Here's how the part is built. I have some questions about the finished solid (model axes, mm). A direction names the side the tool comes from. Round coordinates to 2 decimals unless told otherwise and drop trailing zeros. Order: outer loops, then holes, each group sorted by start corner. A loop starts at its lowest first (then second) coordinate and runs counter-clockwise, first axis right, second up.
```python
from build123d import *

# Parameters (mm, degrees)
F1_DEPTH  = 40
F2_R      = 5
F3_R      = 2.15
F4_DEPTH  = 25
F5_W      = 4.5
F5_H      = 10
F6_DEPTH  = 58.601
F7_R      = 2.24999
F8_W      = 40
F8_H      = 21.2
F9_DEPTH  = 2.4
F10_W     = 40
F10_H     = 21.2
F11_DEPTH = 2.4
F12_W     = 4.3
F12_H     = 9.6518629789
F13_DEPTH = 10


# Not quite as in the source:
# - a fillet or chamfer is up to 0.001 mm smaller than in the source, because OpenCascade refuses the exact size


with BuildPart() as f1:
    # F0 (on Front) → F1 (new body)
    with BuildSketch(Plane.XZ):
        Polygon((25.3, -18.75), (29.3, -18.75), (29.3, 18.75), (-29.3, 18.75), (-29.3, -18.75), (-25.3, -18.75), (-25.3, 14.75), (25.3, 14.75), align=None)
    extrude(amount=F1_DEPTH)

    # F2
    f2_edges = [f1.edges().sort_by_distance(p)[0] for p in [
        (-29.3, -20, 18.75),
        (29.3, -20, 18.75),
    ]]
    fillet(f2_edges, radius=F2_R)

    # F3 (on face) → F4 (cut)
    with BuildSketch(Plane.XY.offset(18.75)):
        with Locations((0, -20)):
            Circle(F3_R)
    extrude(amount=-F4_DEPTH, mode=Mode.SUBTRACT)

    # F5 (on face) → F6 (cut, through all)
    with BuildSketch(Plane.YZ.offset(29.3)):
        with Locations((-20, -9.25)):
            Rectangle(F5_W, F5_H)
    extrude(amount=-F6_DEPTH, mode=Mode.SUBTRACT)

    # F7 (radius 2.25 in the source; OpenCascade refuses exactly that, so slightly less here)
    f7_edges = [f1.edges().sort_by_distance(p)[0] for p in [
        (27.3, -17.75, -4.25),
        (27.3, -22.25, -4.25),
        (27.3, -17.75, -14.25),
        (27.3, -22.25, -14.25),
        (-27.3, -17.75, -4.25),
        (-27.3, -17.75, -14.25),
        (-27.3, -22.25, -4.25),
        (-27.3, -22.25, -14.25),
    ]]
    fillet(f7_edges, radius=F7_R)

    # F8 (on face) → F9 (join)
    with BuildSketch(Plane(origin=(25.3, 0, 0), x_dir=(0, -1, 0), z_dir=(-1, 0, 0))):
        with Locations((20, -8.15)):
            Rectangle(F8_W, F8_H)
        with BuildLine():
            ThreePointArc((17.75, -6.5), (20, -4.25), (22.25, -6.5))
            Line((22.25, -6.5), (22.25, -12))
            ThreePointArc((22.25, -12), (20, -14.25), (17.75, -12))
            Line((17.75, -12), (17.75, -6.5))
        make_face(mode=Mode.SUBTRACT)
    extrude(amount=F9_DEPTH)

    # F10 (on face) → F11 (join)
    with BuildSketch(Plane.YZ.offset(-25.3)):
        with Locations((-20, -8.15)):
            Rectangle(F10_W, F10_H)
        with BuildLine():
            ThreePointArc((-22.25, -6.5), (-20, -4.25), (-17.75, -6.5))
            Line((-17.75, -6.5), (-17.75, -12))
            ThreePointArc((-17.75, -12), (-20, -14.25), (-22.25, -12))
            Line((-22.25, -12), (-22.25, -6.5))
        make_face(mode=Mode.SUBTRACT)
    extrude(amount=F11_DEPTH)

    # F12 (on face) → F13 (join)
    with BuildSketch(Plane(origin=(0, 0, 14.75), x_dir=(1, 0, 0), z_dir=(0, 0, -1))):
        with Locations((0, 35.1740685105)):
            Rectangle(F12_W, F12_H)
    extrude(amount=F13_DEPTH)


solid = f1.part
```
1) If we section it at D-D (z = 8.5): Write out the boundary of the cut face in (x, y), plus the area to 3 significant figures.
2) If we section it at B-B (z = -10.5): Write out the boundary of the cut face in (x, y).
3) We'd pull the mould along Y, two halves only. Please class faces 6 (the flat face through (-22.9, -25, -8)), 7 (the cylindrical face through (-0.47, -22.1, 16.78)): +Y half, -Y half, draft (parallel to the pull), parting line (faces both ways), or undercut.
4) I'm going to push flat-ended pins straight in: pin 1 (12 mm diameter, centred on x = 17, z = -5.5, fed in from -Y); pin 2 (1.3 mm diameter, centred on x = 0.5, z = 12, fed in from +Y); pin 3 (4 mm diameter, centred on x = 7, y = -31.5, fed in from -Z); pin 4 (12 mm diameter, centred on x = -4.5, y = -27.5, fed in from -Z). Where does each tip first touch, or does it pass through?
5) I need wall thicknesses on line 1 (X direction, y = -31.5, z = 13); line 2 (X direction, y = -18, z = 1); line 3 (Y direction, x = 0, z = 16). Which ranges of each line are inside material? Lowest first, please.
6) If we section it at C-C (x = 0): Write out the boundary of the cut face in (y, z), plus the area to 3 significant figures.
7) For faces 1 (the flat face through (2.15, -35, 10)), 2 (the flat face through (-26, -20, -18.75)), 3 (the cylindrical face through (-27.33, -21.57, -13.61)), 4 (the cylindrical face through (-27.8, -20.28, 17.32)), 5 (the flat face through (25.3, -20, 9)), which set-ups out of +Z, -Z, +X, -X, +Y, -Y let a thin tool reach every point of the face, with its end or its side?
8) If we section it at A-A (z = -3): Write out the boundary of the cut face in (x, y).
Solutions:
1. outline: (-29.3, -40) - (-25.3, -40) - (-25.3, 0) - (-29.3, 0) - close; (-2.15, -40) - (2.15, -40) - (2.15, -30.35) - (-2.15, -30.35) - close; (25.3, -40) - (29.3, -40) - (29.3, 0) - (25.3, 0) - close
1. area: 362 mm2
2. outline: (-29.3, -40) - (-22.9, -40) - (-22.9, -22.25) - (-29.3, -22.25) - close; (-29.3, -17.75) - (-22.9, -17.75) - (-22.9, 0) - (-29.3, 0) - close; (22.9, -40) - (29.3, -40) - (29.3, -22.25) - (22.9, -22.25) - close; (22.9, -17.75) - (29.3, -17.75) - (29.3, 0) - (22.9, 0) - close
3. face 6: draft
3. face 7: undercut
4. pin 1: stops at y = -40
4. pin 2: stops at y = -30.35
4. pin 3: stops at z = 14.75
4. pin 4: stops at z = 4.75
5. line 1: x = -29.3 to -25.3, -2.15 to 2.15, 25.3 to 29.3
5. line 2: x = -29.3 to -22.9, 22.9 to 29.3
5. line 3: y = -40 to -22.15, -17.85 to 0
6. outline: (-40, 4.75) - (-30.35, 4.75) - (-30.35, 14.75) - (-22.15, 14.75) - (-22.15, 18.75) - (-40, 18.75) - close; (-17.85, 14.75) - (0, 14.75) - (0, 18.75) - (-17.85, 18.75) - close
6. area: 239 mm2
7. face 1: -Z, +Y, -Y
7. face 2: -Z, +X, -X, +Y, -Y
7. face 3: +X, -X
7. face 4: +Z, -X, +Y, -Y
7. face 5: +Y, -Y
8. outline: (-29.3, -40) - (-22.9, -40) - (-22.9, 0) - (-29.3, 0) - close; (22.9, -40) - (29.3, -40) - (29.3, 0) - (22.9, 0) - close
